from build123d import *

# Parameters (mm, degrees)
ESBO_O1_W                = 40
ESBO_O1_H                = 15.5
RESSALTO_EXTRUS_O1_DEPTH = 30
ESBO_O2_W                = 7
ESBO_O2_H                = 7
CORTE_EXTRUS_O1_DEPTH    = 12
ESBO_O5_W                = 40
ESBO_O5_H                = 45
RESSALTO_EXTRUS_O2_DEPTH = 5
ESBO_O6_W                = 40
ESBO_O6_H                = 15.5
RESSALTO_EXTRUS_O3_DEPTH = 25
ESBO_O7_W                = 40
ESBO_O7_H                = 45
RESSALTO_EXTRUS_O4_DEPTH = 5
ESBO_O8_R                = 4
CORTE_EXTRUS_O2_DEPTH    = 89.600225733


with BuildPart() as part:
    # Esboço1 → Ressalto-extrusão1 (new body)
    with BuildSketch(Plane(origin=(0, 0, 0), x_dir=(1, 0, 0), z_dir=(0, 1, 0))):
        with Locations((20, 7.75)):
            Rectangle(ESBO_O1_W, ESBO_O1_H)
    extrude(amount=RESSALTO_EXTRUS_O1_DEPTH)

    # Esboço2 → Corte-extrusão1 (cut)
    with BuildSketch(Plane.XZ):
        with Locations((7.5, -7.5)):
            Rectangle(ESBO_O2_W, ESBO_O2_H)
        with Locations((32.5, -7.5)):
            Rectangle(ESBO_O2_W, ESBO_O2_H)
    extrude(amount=-CORTE_EXTRUS_O1_DEPTH, mode=Mode.SUBTRACT)

    # Esboço5 → Ressalto-extrusão2 (add)
    with BuildSketch(Plane(origin=(0, 30, 0), x_dir=(1, 0, 0), z_dir=(0, 1, 0))):
        with Locations((20, 22.5)):
            Rectangle(ESBO_O5_W, ESBO_O5_H)
    extrude(amount=RESSALTO_EXTRUS_O2_DEPTH)

    # Esboço6 → Ressalto-extrusão3 (add)
    with BuildSketch(Plane(origin=(0, 35, 0), x_dir=(1, 0, 0), z_dir=(0, 1, 0))):
        with Locations((20, 7.75)):
            Rectangle(ESBO_O6_W, ESBO_O6_H)
    extrude(amount=RESSALTO_EXTRUS_O3_DEPTH)

    # Esboço7 → Ressalto-extrusão4 (add)
    with BuildSketch(Plane(origin=(0, 60, 0), x_dir=(1, 0, 0), z_dir=(0, 1, 0))):
        with Locations((20, 22.5)):
            Rectangle(ESBO_O7_W, ESBO_O7_H)
    extrude(amount=RESSALTO_EXTRUS_O4_DEPTH)

    # Esboço8 → Corte-extrusão2 (cut, through all)
    with BuildSketch(Plane(origin=(0, 65, 0), x_dir=(1, 0, 0), z_dir=(0, 1, 0))):
        with Locations(Location((20, 38.5, 0), (0, 0, 270))):
            Circle(ESBO_O8_R)
    extrude(amount=-CORTE_EXTRUS_O2_DEPTH, mode=Mode.SUBTRACT)


solid = part.part
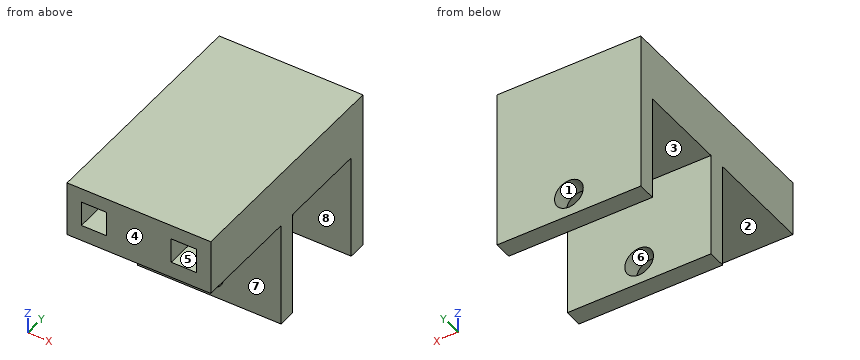
Geometry: final body of the model. Coordinates: model frame, mm. Face numbers are marked on the shaded views. A direction names the side the tool comes from. Coordinates: 2 decimals unless noted, no trailing zeros. Order: outer loops, then holes, each group sorted by start corner. A loop starts at its lowest first (then second) coordinate and runs counter-clockwise, first axis right, second up.
(1) Section query A-A (z = -18.5). Return the cut outline in (x, y), plus the area to 3 significant figures.
(2) Section query D-D (x = 31). Return the cut outline in (y, z).
(3) Section query C-C (z = -38.5). Return the cut outline in (x, y), plus the area to 3 significant figures.
(4) First-contact query: pin 1 (5.5 mm diameter, centred on x = 32, z = -8, fed in from -Y); pin 2 (5.5 mm diameter, centred on x = 33.5, y = 4.5, fed in from -Z); pin 3 (9 mm diameter, centred on x = 20, z = -38.5, fed in from -Y). Flat tips, straight axial feed; report the tip coordinate or a pass-through.
(5) Draft query along Y for the marked faces 6, 7 and 8. Return one class per face: pulls with the +Y half, pulls with the -Y half, needs draft (parallel to the pull), parting line crosses it, or undercut.
(6) Access query for the marked faces 1, 2, 3, 4 and 5. Directions: +Z, -Z, +X, -X, +Y, -Y. A direction counts if a zero-diameter tool reaches every point of the face in a straight line with its end or side. Return the directions, or none.
(7) Material intervals for probe 1 along Y at (x, z) = (13.5, -28.5); probe 2 along X at (y, z) = (31.35, -38.5); probe 3 along Z at (x, y) = (4.5, 20.5), sorted ascending.
(8) Section query B-B (x = 20). Return the cut outline in (y, z), plus the area to 3 significant figures.
Solution:
1. outline: (0, 30) - (40, 30) - (40, 35) - (0, 35) - close; (0, 60) - (40, 60) - (40, 65) - (0, 65) - close
1. area: 400 mm2
2. outline: (0, -15.5) - (30, -15.5) - (30, -45) - (35, -45) - (35, -15.5) - (60, -15.5) - (60, -45) - (65, -45) - (65, 0) - (0, 0) - (0, -4) - (12, -4) - (12, -11) - (0, -11) - close
3. outline: (0, 30) - (16, 30) - (16, 35) - (0, 35) - close; (0, 60) - (16, 60) - (16, 65) - (0, 65) - close; (24, 30) - (40, 30) - (40, 35) - (24, 35) - close; (24, 60) - (40, 60) - (40, 65) - (24, 65) - close
3. area: 320 mm2
4. pin 1: stops at y = 12
4. pin 2: stops at z = -15.5
4. pin 3: stops at y = 30
5. face 6: needs draft
5. face 7: pulls with the -Y half
5. face 8: undercut
6. face 1: +Y, -Y
6. face 2: -Z, +X, -X, -Y
6. face 3: -Z, +X, -X
6. face 4: +Z, -Z, +X, -X, -Y
6. face 5: -Y
7. probe 1: y = 30 to 35, 60 to 65
7. probe 2: x = 0 to 16, 24 to 40
7. probe 3: z = -15.5 to 0
8. outline: (0, -15.5) - (30, -15.5) - (30, -34.5) - (35, -34.5) - (35, -15.5) - (60, -15.5) - (60, -34.5) - (65, -34.5) - (65, 0) - (0, 0) - close; (30, -45) - (35, -45) - (35, -42.5) - (30, -42.5) - close; (60, -45) - (65, -45) - (65, -42.5) - (60, -42.5) - close
8. area: 1,220 mm2
